Input: part model. Units: mm. Frame: model coordinates. A direction names the side the tool comes from. Coordinates: 2 decimals unless noted, no trailing zeros. Order: outer loops, then holes, each group sorted by start corner. A loop starts at its lowest first (then second) coordinate and runs counter-clockwise, first axis right, second up. Notation, with made-up numbers: (-2.5, -15.5) -> (51.5, -15.5) arc R22 ccw to (51.5, 5.5) -> close; hole circle Ø8 at (57.5, 37.5). An arc over 180 degrees is marked (long way). Write each question's results on one line, items separated by ' | '.
Autodesk Inventor part; units mm, degrees
ref_plane "shroud_to_body_XY" through (0, 0, 0) normal (0, 1, 0) x (1, 0, 0)
ref_plane "shroud_to_body_YZ" through (0, 0, 0) normal (1, 0, 0) x (0, 0, -1)
ref_plane "shroud_to_body_ZX" through (0, 0, 0) normal (0, 0, -1) x (0, 1, 0)
sketch "Sketch_1" plane through (0, 0, 0) normal (0, 1, 0) x (-1, 0, 0)
  line L0 (6.5024, 3.9497) -> (-6.5024, 3.9497)
  line L1 (-6.5024, 3.9497) -> (-6.5024, -3.9497)
  line L2 (-6.5024, -3.9497) -> (6.5024, -3.9497)
  line L3 (6.5024, -3.9497) -> (6.5024, 3.9497)
extrude "Extrusion1" add sketch "Sketch_1" along normal blind 0.2032
sketch "Sketch_2" plane through (0, 0, -3.9497) normal (0, 0, 1) x (1, 0, 0)
  line L0 (-6.0389, -6.018) -> (-3.1581, -6.018)
  line L1 (-3.1581, -6.018) -> (-3.1581, -6.4159)
  arc A0 (-3.1581, -6.4159) -> (-1.9219, -6.4159) centre (-2.54, -6.4159) ccw
  line L2 (-1.9219, -6.4159) -> (-1.9219, -6.018)
  line L3 (-1.9219, -6.018) -> (1.9219, -6.018)
  line L4 (1.9219, -6.018) -> (1.9219, -6.4159)
  arc A1 (1.9219, -6.4159) -> (3.1581, -6.4159) centre (2.54, -6.4159) ccw
  line L5 (3.1581, -6.4159) -> (3.1581, -6.018)
  line L6 (3.1581, -6.018) -> (6.0389, -6.018)
  line L7 (6.0389, -6.018) -> (6.0389, 0)
  line L8 (6.0389, 0) -> (-6.0389, 0)
  line L9 (-6.0389, 0) -> (-6.0389, -6.018)
extrude "Extrusion2" add sketch "Sketch_2" along normal blind 0.2032
sketch "Sketch_3" plane through (0, 0, 3.9497) normal (0, 0, 1) x (1, 0, 0)
  line L0 (-6.0389, -6.018) -> (-3.1581, -6.018)
  line L1 (-3.1581, -6.018) -> (-3.1581, -6.4159)
  arc A0 (-3.1581, -6.4159) -> (-1.9219, -6.4159) centre (-2.54, -6.4159) ccw
  line L2 (-1.9219, -6.4159) -> (-1.9219, -6.018)
  line L3 (-1.9219, -6.018) -> (1.9219, -6.018)
  line L4 (1.9219, -6.018) -> (1.9219, -6.4159)
  arc A1 (1.9219, -6.4159) -> (3.1581, -6.4159) centre (2.54, -6.4159) ccw
  line L5 (3.1581, -6.4159) -> (3.1581, -6.018)
  line L6 (3.1581, -6.018) -> (6.0389, -6.018)
  line L7 (6.0389, -6.018) -> (6.0389, 0)
  line L8 (6.0389, 0) -> (-6.0389, 0)
  line L9 (-6.0389, 0) -> (-6.0389, -6.018)
extrude "Extrusion3" add sketch "Sketch_3" against normal blind 0.2032
ref_plane "shroud_to_body_XY" through (0, 0, 0) normal (0, 1, 0) x (1, 0, 0)
ref_plane "shroud_to_body_YZ" through (0, 0, 0) normal (1, 0, 0) x (0, 0, -1)
ref_plane "shroud_to_body_ZX" through (0, 0, 0) normal (0, 0, -1) x (0, 1, 0)
properties part number "M20_ang_t_shorud1230TX-switch"
(1) Reachability of faces 1 (the face through (0, -3, 3.746)), 2 (the face through (0, -3, -3.95)) from +Z, -Z, +X, -X, +Y, -Y: full face, straight path, thin tool, end or side. Return the list, or none.
Return value:
face 1: +X, -X, -Y | face 2: -Z, +X, -X, +Y, -Y
(2) Line query: line 1 along Z through (x, y) = (5, -2.5); line 2 along Y through (x, z) = (-5, 0). Output: solid intervals per line, ascending. Write a range as from..to.
Return value:
line 1: -3.95..-3.75, 3.75..3.95 | line 2: 0..0.2
(3) Cut plane C-C, the plane y = -3. Return loops of the section in (x, z).
Return value:
outline: (-6.04, -3.95) -> (6.04, -3.95) -> (6.04, -3.75) -> (-6.04, -3.75) -> close; (-6.04, 3.75) -> (6.04, 3.75) -> (6.04, 3.95) -> (-6.04, 3.95) -> close
(4) Cut plane B-B, the plane x = 2.54. Return loops of the section in (y, z), plus the area to 3 significant figures.
Return value:
outline: (-7.03, -3.95) -> (0.2, -3.95) -> (0.2, 3.95) -> (-7.03, 3.95) -> (-7.03, 3.75) -> (0, 3.75) -> (0, -3.75) -> (-7.03, -3.75) -> close | area: 4.46 mm2
(5) Cut plane A-A, the plane y = -6.25. Return loops of the section in (x, z).
Return value:
outline: (-3.16, -3.95) -> (-1.92, -3.95) -> (-1.92, -3.75) -> (-3.16, -3.75) -> close; (-3.16, 3.75) -> (-1.92, 3.75) -> (-1.92, 3.95) -> (-3.16, 3.95) -> close; (1.92, -3.95) -> (3.16, -3.95) -> (3.16, -3.75) -> (1.92, -3.75) -> close; (1.92, 3.75) -> (3.16, 3.75) -> (3.16, 3.95) -> (1.92, 3.95) -> close
(6) Pin query (flat end, axial travel): P1, Ø1.5, axis at y = -4.5, z = 2, coming from the +X side; P2, Ø2.5, axis at x = -0.5, z = 2, coming from the -Y side; P3, Ø3, axis at y = -2.5, z = 3, coming from the +X side. Return the tip coordinate at first contact, or that it passes through.
Return value:
P1: through | P2: y = 0 | P3: x = 6.04
(7) Cut plane D-D, the plane z = 2.5. Return loops of the section in (x, y), plus the area to 3 significant figures.
Return value:
outline: (-6.5, 0) -> (6.5, 0) -> (6.5, 0.2) -> (-6.5, 0.2) -> close | area: 2.64 mm2
(8) Mould query, pull axis Z, two halves, no side actions, for faces 3 (the face through (0, -3, 3.95)), 4 (the face through (0, 0, 0)), 5 (the face through (0, 0.203, 0)). Classes: +Z half, -Z half, draft (parallel to the pull), parting line (faces both ways), or undercut.
Return value:
face 3: +Z half | face 4: undercut | face 5: draft
